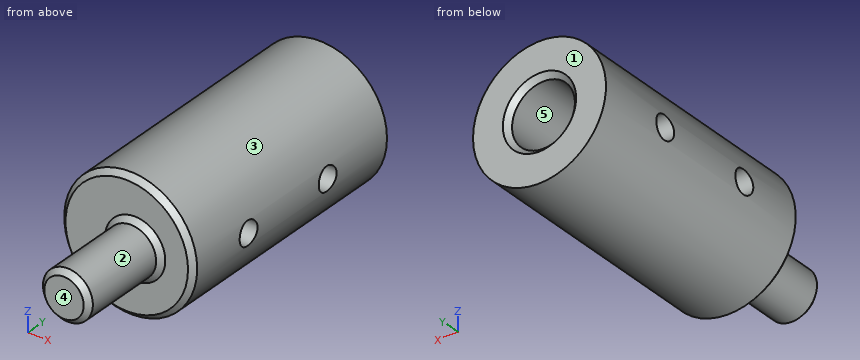
from build123d import *

# Parameters (mm, degrees)
SKETCH1_R             = 6.35
BOSS_EXTRUDE1_DEPTH   = 24.5
SKETCH2_R             = 3
CUT_EXTRUDE1_DEPTH    = 21.6
F_4_40_TAPPED_HOLE1_D = 2.2606
SKETCH5_R             = 2.38125
BOSS_EXTRUDE2_DEPTH   = 9
CHAMFER2_SIZE         = 0.5


with BuildPart() as part:
    # Sketch1 → Boss-Extrude1 (new body)
    with BuildSketch(Plane(origin=(0, 0, 0), x_dir=(1, 0, 0), z_dir=(0, 1, 0))):
        Circle(SKETCH1_R)
    extrude(amount=BOSS_EXTRUDE1_DEPTH)

    # Sketch2 → Cut-Extrude1 (cut)
    with BuildSketch(Plane(origin=(0, 24.5, 0), x_dir=(1, 0, 0), z_dir=(0, 1, 0))):
        Circle(SKETCH2_R)
    extrude(amount=-CUT_EXTRUDE1_DEPTH, mode=Mode.SUBTRACT)

    # #4-40 Tapped Hole1 (through all)
    with Locations(Plane(origin=(6.35, 0, 0), x_dir=(0, 0, -1), z_dir=(1, 0, 0))):
        with Locations((0, 17), (0, 7)):
            Hole(F_4_40_TAPPED_HOLE1_D / 2)

    # Sketch5 → Boss-Extrude2 (add)
    with BuildSketch(Plane(origin=(0, 0, 0), x_dir=(-1, 0, 0), z_dir=(0, -1, 0))):
        with Locations((-0.8, 0)):
            Circle(SKETCH5_R)
    extrude(amount=BOSS_EXTRUDE2_DEPTH)

    # Chamfer2
    chamfer2_edges = [part.edges().sort_by_distance(p)[0] for p in [
        (-6.35, 0, 0),
        (3.18125, 0, 0),
        (3.18125, -9, 0),
        (-3, 24.5, 0),
    ]]
    chamfer(chamfer2_edges, length=CHAMFER2_SIZE)


solid = part.part
For this review, take the finished solid that the model builds, in its own axes (mm). Face numbers are marked on the shaded views. A direction names the side the tool comes from. Round coordinates to 2 decimals unless told otherwise and drop trailing zeros. Write each loop counter-clockwise with the first axis right and the second up, starting at its lowest first coordinate (ties: lowest second). Pieces come first, ordered by that corner, then holes. Notation, with made-up numbers: (88.25, -4.5) - (92.25, -4.5) arc R16 cw to (92.25, 18.5) - close; hole circle Ø7 at (4.25, 12.25). An arc over 180 degrees is marked (long way). Use a Markdown table: item, result.
Q1. Machinability: for the marked faces 1 and 2, which of the approach directions +Z, -Z, +X, -X, +Y, -Y give a long, thin tool a straight path to every point of the face, cutting with its end or side? Answer none if there is none.
Derived:
| item | result |
|---|---|
| face 1 | +Z, -Z, +X, -X, +Y |
| face 2 | -Y |
Q2. We need section B-B (y = 17). Give the boundary of the cut face in (x, z), plus the area to 3 significant figures.
Derived:
| item | result |
|---|---|
| outline | (-6.25, -1.13) arc R6.35 ccw to (6.25, -1.13) - (2.78, -1.13) arc R3 cw to (-2.78, -1.13) - close; (-6.25, 1.13) - (-2.78, 1.13) arc R3 cw to (2.78, 1.13) - (6.25, 1.13) arc R6.35 ccw to start |
| area | 83.1 mm2 |
Q3. The part is to be moulded in two halves that separate along Z. For the marked faces 3, 4 and 5, say which applies: pulls with the +Z half, pulls with the -Z half, needs draft (parallel to the pull), parting line crosses it, or undercut.
Derived:
| item | result |
|---|---|
| face 3 | parting line crosses it |
| face 4 | needs draft |
| face 5 | undercut |
Q4. Clearance check with flat-ended pins moving along their axes: pin 1 (2.5 mm diameter, centred on y = 7, z = 0, fed in from +X); pin 2 (1.5 mm diameter, centred on y = 3.5, z = 3, fed in from -X); pin 3 (4 mm diameter, centred on x = -3, y = 4, fed in from +Z); pin 4 (1.5 mm diameter, centred on y = 6, z = -2, fed in from -X). State where each tip first meets the part, or that it passes through.
Derived:
| item | result |
|---|---|
| pin 1 | stops at x = 6.35 |
| pin 2 | stops at x = -5.94 |
| pin 3 | stops at z = 6.27 |
| pin 4 | stops at x = -6.23 |
Q5. Wall thickness on line 1 along Y through (x, z) = (4.8, 0); line 2 along Y through (x, z) = (-4.25, 2.5); line 3 along Z through (x, y) = (-5.3, 7): over which ranges is each line inside the solid? List them lowest first.
Derived:
| item | result |
|---|---|
| line 1 | y = 0 to 5.87, 8.13 to 15.87, 18.13 to 24.5 |
| line 2 | y = 0 to 24.5 |
| line 3 | z = -3.5 to -1.13, 1.13 to 3.5 |
Q6. We need section C-C (y = 4). Give the boundary of the cut face in (x, z).
Derived:
| item | result |
|---|---|
| outline | circle Ø12.7 at (0, 0); hole circle Ø6 at (0, 0) |
Q7. We need section A-A (z = 0). State how many separate pieces and enclosed holes the cut face has, plus the area to 3 significant figures.
Derived:
| item | result |
|---|---|
| separate pieces | 5 |
| enclosed holes | 0 |
| area | 194 mm2 |
